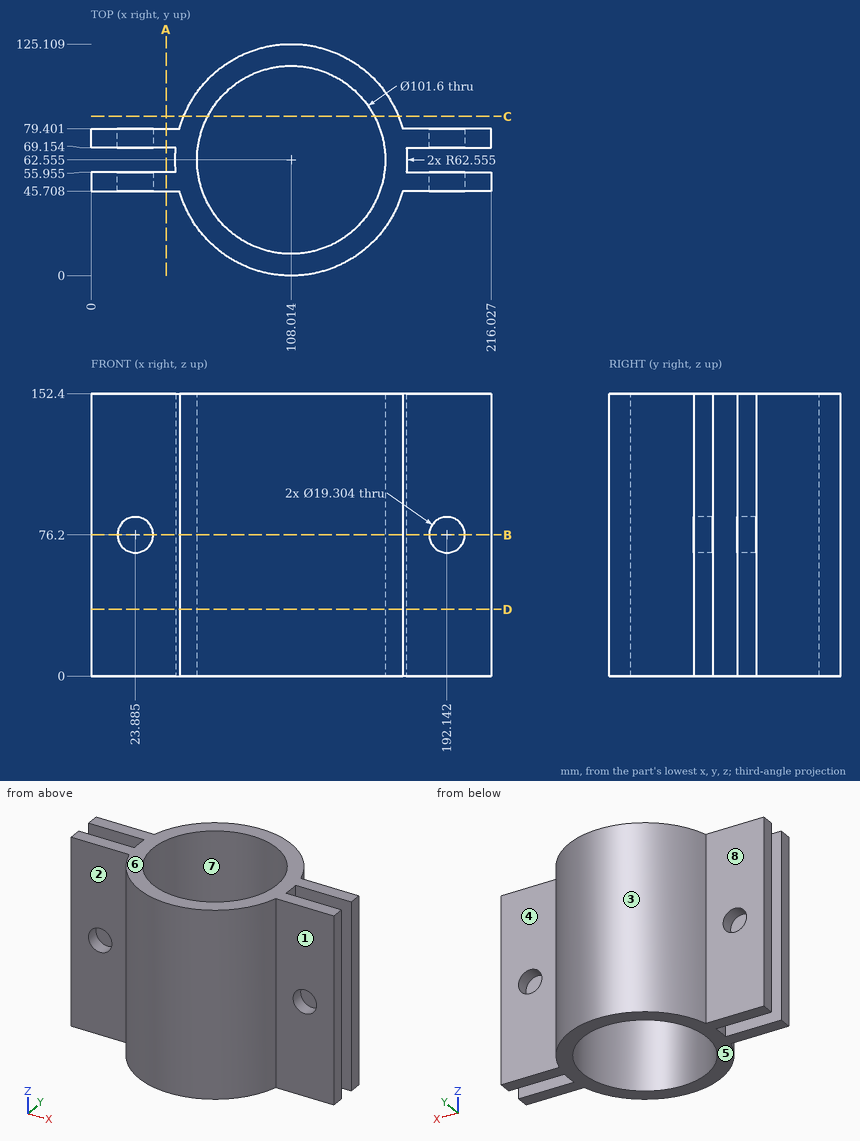
Drawing for the job (mm, zero at the part's lowest x, y, z). A direction names the side the tool comes from. Give positions to 0.01 mm unless a question says otherwise; leave off trailing zeros. Order: outer loops, then holes, each group sorted by start corner. A loop starts at its lowest first (then second) coordinate and runs counter-clockwise, first axis right, second up. Notation, with made-up numbers: M -24.75,82.5 L 28.25,82.5 A20 cw 28.25,118.5 Z; hole C 83.25,5.25 d4. An arc over 180 degrees is marked long. Put each result on its own line as item: value.
Item 1: 3-axis set-ups, long thin cutter, end or side, ignore diameter. For the marked faces 1, 2, 3, 4 and 5: which of +Z, -Z, +X, -X, +Y, -Y reach the whole face in a straight line?
From the geometry:
face 1: +Z, -Z, +X, -Y
face 2: +Z, -Z, -X, -Y
face 3: +Z, -Z, +Y
face 4: +Z, -Z, +X, +Y
face 5: -Z, +X, -X, +Y, -Y
Item 2: Slice it at B-B, the plane z = 76.2. Give the number of separate pieces and of enclosed holes in the cut face, plus the area to 3 significant figures.
From the geometry:
separate pieces: 5
enclosed holes: 1
area: 5,310 mm2
Item 3: Flat gauge pins, fed straight in: pin 1 Ø1 at (y, z) = (58, 40) entering from -X; pin 2 Ø13.5 at (x, z) = (15.5, 52.5) entering from +Y; pin 3 Ø24 at (x, z) = (28, 60.5) entering from -Y; pin 4 Ø8 at (y, z) = (44, 66) entering from +X. Where does each tip first touch, or does it go through?
From the geometry:
pin 1: stops at x = 45.59
pin 2: stops at y = 79.4
pin 3: stops at y = 45.71
pin 4: stops at x = 216.03
Item 4: Two-plate mould, pull along Y, no slides. Class the marked faces 6, 7 and 8: +Y half, -Y half, draft (parallel to the pull), parting line (faces both ways), or undercut.
From the geometry:
face 6: draft
face 7: undercut
face 8: +Y half
Item 5: Slice it at D-D, the plane z = 36. Write the cut outline in (x, y) (1 decimal), plus the area to 3 significant figures.
From the geometry:
outline: M 0,45.7 L 47.8,45.7 A62.6 ccw 168.3,45.7 L 216,45.7 L 216,56 L 170.2,56 A62.6 ccw 170.2,69.2 L 216,69.2 L 216,79.4 L 168.3,79.4 A62.6 ccw 47.8,79.4 L 0,79.4 L 0,69.2 L 45.8,69.2 A62.6 ccw 45.8,56 L 0,56 Z; hole C 108,62.6 d101.6
area: 6,100 mm2
Item 6: Slice it at A-A, the plane x = 40.5. Write the cut outline in (y, z) (1 decimal).
From the geometry:
outline: M 45.7,0 L 56,0 L 56,152.4 L 45.7,152.4 Z; M 69.2,0 L 79.4,0 L 79.4,152.4 L 69.2,152.4 Z
Item 7: Probe line 1 (Y direction, x = 19.5, z = 98) (1 decimal); line 2 (X direction, y = 62, z = 141) (1 decimal). List the from-to ranges inside material, lowest first. Write a range as [from, to].
From the geometry:
line 1: y = [45.7, 56], [69.2, 79.4]
line 2: x = [45.5, 57.2], [158.8, 170.6]
Item 8: Slice it at C-C, the plane y = 86. Write the cut outline in (x, z).
From the geometry:
outline: M 50.02,0 L 62.95,0 L 62.95,152.4 L 50.02,152.4 Z; M 153.08,0 L 166.01,0 L 166.01,152.4 L 153.08,152.4 Z
